```python
from build123d import *

# Parameters (mm, degrees)
SKETCH1_R           = 3.2004
SKETCH1_R_2         = 2.159
SKETCH1_W           = 3.3274
SKETCH1_H           = 6.5024
BOSS_EXTRUDE1_DEPTH = 3.175
FILLET1_R           = 6.35
CUT_EXTRUDE1_DEPTH  = 119.620638985
CUT_EXTRUDE2_DEPTH  = 119.620638985


with BuildPart() as part:
    # Sketch1 → Boss-Extrude1 (new body)
    with BuildSketch(Plane(origin=(0, 0, 0), x_dir=(1, 0, 0), z_dir=(0, 1, 0))):
        with BuildLine():
            Line((46.403243059, 26.253216793), (50.58203093, 29.139941438))
            Line((50.58203093, 29.139941438), (50.810401684, 29.296808651))
            ThreePointArc((50.810401684, 29.296808651), (52.903191273, 29.710570717), (54.573236871, 28.38319925))
            ThreePointArc((54.573236871, 28.38319925), (57.812038803, 18.519910789), (58.021057072, 8.140575136))
            ThreePointArc((58.021057072, 8.140575136), (58.019631397, 7.454008247), (58.110797015, 6.773519483))
            ThreePointArc((58.110797015, 6.773519483), (77.605374828, -7.708974753), (90.50576443, 12.866767069))
            ThreePointArc((90.50576443, 12.866767069), (43.472529066, 70.626376988), (-30.323774881, 60.506925891))
            ThreePointArc((-30.323774881, 60.506925891), (-30.739824891, 60.355496072), (-31.123258654, 60.134120485))
            Line((-31.123258654, 60.134120485), (-48.980521588, 47.630330367))
            ThreePointArc((-48.980521588, 47.630330367), (-49.319688664, 47.345735399), (-49.604283632, 47.006568323))
            Line((-49.604283632, 47.006568323), (-56.690646192, 36.886193758))
            ThreePointArc((-56.690646192, 36.886193758), (-57.032441055, 36.19310234), (-57.15, 35.429309609))
            Line((-57.15, 35.429309609), (-57.15, 35.009609836))
            ThreePointArc((-57.15, 35.009609836), (-56.859279722, 33.82963495), (-56.053668716, 32.919772369))
            Line((-56.053668716, 32.919772369), (-50.58203093, 29.139941438))
            Line((-50.58203093, 29.139941438), (-46.403243059, 26.253216793))
            Line((-46.403243059, 26.253216793), (0, -5.80234322))
            Line((0, -5.80234322), (46.403243059, 26.253216793))
        make_face()
        with Locations(Location((0, 0, 0), (0, 0, 270))):
            Circle(SKETCH1_R, mode=Mode.SUBTRACT)
        with Locations(Location((-14.172189073, 49.146835797, 0), (0, 0, 270))):
            Circle(SKETCH1_R_2, mode=Mode.SUBTRACT)
        with Locations(Location((-8.088821086, 24.747779464, 0), (0, 0, 90))):
            Circle(SKETCH1_R_2, mode=Mode.SUBTRACT)
        with Locations(Location((-34.819826997, 37.519095065, 0), (0, 0, 270))):
            Circle(SKETCH1_R_2, mode=Mode.SUBTRACT)
        with Locations(Location((-19.338403539, 17.703776655, 0), (0, 0, 90))):
            Circle(SKETCH1_R_2, mode=Mode.SUBTRACT)
        with Locations(Location((34.819826997, 37.519095065, 0), (0, 0, 90))):
            Circle(SKETCH1_R_2, mode=Mode.SUBTRACT)
        with Locations(Location((19.338403539, 17.703776655, 0), (0, 0, 270))):
            Circle(SKETCH1_R_2, mode=Mode.SUBTRACT)
        with Locations(Location((8.088821086, 24.747779464, 0), (0, 0, 270))):
            Circle(SKETCH1_R_2, mode=Mode.SUBTRACT)
        with Locations(Location((14.172189073, 49.146835797, 0), (0, 0, 90))):
            Circle(SKETCH1_R_2, mode=Mode.SUBTRACT)
        Polygon((-14.194632296, 62.360921096), (-20.479237716, 60.793992979), (-18.912309598, 54.50938756), (-12.627704179, 56.076315677), align=None, mode=Mode.SUBTRACT)
        Polygon((-3.471928118, 19.354503621), (-9.756533537, 17.787575503), (-8.189605419, 11.502970084), (-1.905, 13.069898202), align=None, mode=Mode.SUBTRACT)
        Polygon((-12.927019028, 14.654633554), (-18.030964679, 10.666994178), (-14.043325303, 5.563048527), (-8.939379652, 9.550687903), align=None, mode=Mode.SUBTRACT)
        Polygon((-36.227343223, 44.477688535), (-41.331288874, 40.490049159), (-45.31892825, 45.59399481), (-40.214982599, 49.581634186), align=None, mode=Mode.SUBTRACT)
        Polygon((40.214982599, 49.581634186), (45.31892825, 45.59399481), (41.331288874, 40.490049159), (36.227343223, 44.477688535), align=None, mode=Mode.SUBTRACT)
        Polygon((8.939379652, 9.550687903), (14.043325303, 5.563048527), (18.030964679, 10.666994178), (12.927019028, 14.654633554), align=None, mode=Mode.SUBTRACT)
        Polygon((9.756533537, 17.787575503), (8.189605419, 11.502970084), (1.905, 13.069898202), (3.471928118, 19.354503621), align=None, mode=Mode.SUBTRACT)
        Polygon((14.194632296, 62.360921096), (12.627704179, 56.076315677), (18.912309598, 54.50938756), (20.479237716, 60.793992979), align=None, mode=Mode.SUBTRACT)
        with Locations((63.088721213, 9.69176707)):
            Rectangle(SKETCH1_W, SKETCH1_H, mode=Mode.SUBTRACT)
    extrude(amount=BOSS_EXTRUDE1_DEPTH)

    # Fillet1
    fillet1_edges = [part.edges().sort_by_distance(p)[0] for p in [
        (0, 1.5875, 5.80234322),
    ]]
    fillet(fillet1_edges, radius=FILLET1_R)

    # Sketch2 → Cut-Extrude1 (cut, through all)
    with BuildSketch(Plane(origin=(0, 3.175, 0), x_dir=(1, 0, 0), z_dir=(0, 1, 0))):
        with BuildLine():
            ThreePointArc((87.135212516, 5.657351319), (81.909051328, 31.878788039), (66.223051077, 53.53117591))
            ThreePointArc((66.223051077, 53.53117591), (52.97426357, 52.779767692), (53.725671788, 39.530980185))
            ThreePointArc((53.725671788, 39.530980185), (64.711476112, 24.366572912), (68.371656098, 6.002199057))
            ThreePointArc((68.371656098, 6.002199057), (77.581010438, -3.552003021), (87.135212516, 5.657351319))
        make_face()
    extrude(amount=-CUT_EXTRUDE1_DEPTH, mode=Mode.SUBTRACT)

    # Sketch3 → Cut-Extrude2 (cut, through all)
    with BuildSketch(Plane(origin=(0, 3.175, 0), x_dir=(1, 0, 0), z_dir=(0, 1, 0))):
        with BuildLine():
            ThreePointArc((91.082221145, -2.183816518), (85.424919637, 28.55421491), (68.37898463, 54.750927226))
            ThreePointArc((68.37898463, 54.750927226), (59.749990126, 58.284939929), (51.262155566, 54.424181401))
            ThreePointArc((51.262155566, 54.424181401), (43.754739182, 53.985373594), (36.383549974, 55.4751463))
            ThreePointArc((36.383549974, 55.4751463), (3.225200598, 66.426758828), (-31.123258654, 60.134120485))
            ThreePointArc((-31.123258654, 60.134120485), (64.717904465, 75.405291468), (123.015996485, -2.183816518))
            ThreePointArc((123.015996485, -2.183816518), (86.509258073, -24.398136946), (58.019631397, 7.454008247))
            ThreePointArc((58.019631397, 7.454008247), (71.64980722, -7.317202642), (91.082221145, -2.183816518))
        make_face()
    extrude(amount=-CUT_EXTRUDE2_DEPTH, mode=Mode.SUBTRACT)


solid = part.part
```
Verification items for the finished model (mm, model axes). A direction names the side the tool comes from. Coordinates: 2 decimals unless noted, no trailing zeros. Write each loop counter-clockwise with the first axis right and the second up, starting at its lowest first coordinate (ties: lowest second). Pieces come first, ordered by that corner, then holes. Notation, with made-up numbers: M 58.25,-30 L 107.25,-30 A28 cw 107.25,-1 Z; hole C -26,80 d2. An arc over 180 degrees is marked long. Answer as a JSON object with one key per item and string values. Group by question number.
(1) Gauge pin test, flat ends, axial feed: pin 1 (8 mm diameter, centred on x = 58.5, z = -8, fed in from -Y); pin 2 (1 mm diameter, centred on y = 1.5, z = -11.5, fed in from +X); pin 3 (1 mm diameter, centred on x = 63.5, y = 1.5, fed in from -Z). Record the tip position at first contact, or that the pin passes through.
(2) Material ranges on line 1 (X direction, y = 0.4, z = -60.5); line 2 (X direction, y = 2.55, z = -4.5); line 3 (X direction, y = 1.3, z = -44), recorded low to high.
(3) Cross-section at C-C, the plane z = 0. Record the cut outline in (x, y) (3 decimals), and give its area (3 significant figures).
(4) Tool access check on faces 1 (the face through (10.96, 1.57, -12.14)), 2 (the face through (84.745, 1.61, -30.206)). Record the directions out of +Z, -Z, +X, -X, +Y, -Y that give a thin tool (end or side, any length) a straight path to the whole face; none if there is none.
(5) Cross-section at D-D, the plane y = 2.2. State how many separate pieces and enclosed holes the cut face has, and give its area (3 significant figures).
(6) Cross-section at A-A, the plane x = 0. Record the cut outline in (y, z) (3 decimals), and give its area (3 significant figures).
(7) Release check for a two-part mould opening along Z. For faces 3 (the face through (15, 1.57, -51.14)), 4 (the face through (43.86, 1.61, -53.98)) record: +Z half, -Z half, draft (parallel to the pull), parting line (faces both ways), or undercut.
(8) Cross-section at B-B, the plane z = -24.5. Record the cut outline in (x, y) (1 decimal), and give its area (3 significant figures).
Reply:
{
 "1": {"pin 1": "y = 0", "pin 2": "x = 90.19", "pin 3": "z = -57.89"},
 "2": {"line 1": "-30.31 to -20.41, -13.73 to 13.73, 20.41 to 27.05", "line 2": "-14.91 to 14.91, 58.88 to 68.46, 87.04 to 90.58", "line 3": "-51.71 to -44.07, -36.84 to 36.84, 44.07 to 50.94, 74.91 to 77.2"},
 "3": {"outline": "M -8.399,0 L -3.2,0 L -3.2,3.175 L -8.399,3.175 Z; M 3.2,0 L 8.399,0 L 8.399,3.175 L 3.2,3.175 Z; M 61.293,0 L 70.401,0 L 70.401,3.175 L 61.293,3.175 Z; M 85.106,0 L 88.706,0 L 88.706,3.175 L 85.106,3.175 Z", "area": "73.4 mm²"},
 "4": {"face 1": "+Y, -Y", "face 2": "-Z, +X, +Y, -Y"},
 "5": {"separate pieces": "1", "enclosed holes": "19", "area": "5,140 mm²"},
 "6": {"outline": "M 0,-66.575 L 3.175,-66.575 L 3.175,-3.2 L 0,-3.2 Z; M 0,3.2 L 3.175,3.2 L 3.175,4.435 L 0,4.435 Z", "area": "205 mm²"},
 "7": {"face 3": "undercut", "face 4": "-Z half"},
 "8": {"outline": "M -43.9,0 L -10.2,0 L -10.2,3.2 L -43.9,3.2 Z; M -5.9,0 L 5.9,0 L 5.9,3.2 L -5.9,3.2 Z; M 10.2,0 L 43.9,0 L 43.9,3.2 L 10.2,3.2 Z; M 56.2,0 L 64.7,0 L 64.7,3.2 L 56.2,3.2 Z; M 84.6,0 L 86.9,0 L 86.9,3.2 L 84.6,3.2 Z", "area": "285 mm²"}
}
